Check sheet for the drawn part. Datum: minimum x, y, z corner. Units: mm. Coordinates: 2 decimals unless noted, no trailing zeros. Write each loop counter-clockwise with the first axis right and the second up, starting at its lowest first coordinate (ties: lowest second). Pieces come first, ordered by that corner, then holes. Notation, with made-up numbers: M 12.25,19.25 L 28.25,19.25 A27 cw 28.25,46.25 Z; hole C 79,42 d4. An arc over 180 degrees is marked long. Answer as CSV lines item,"result".
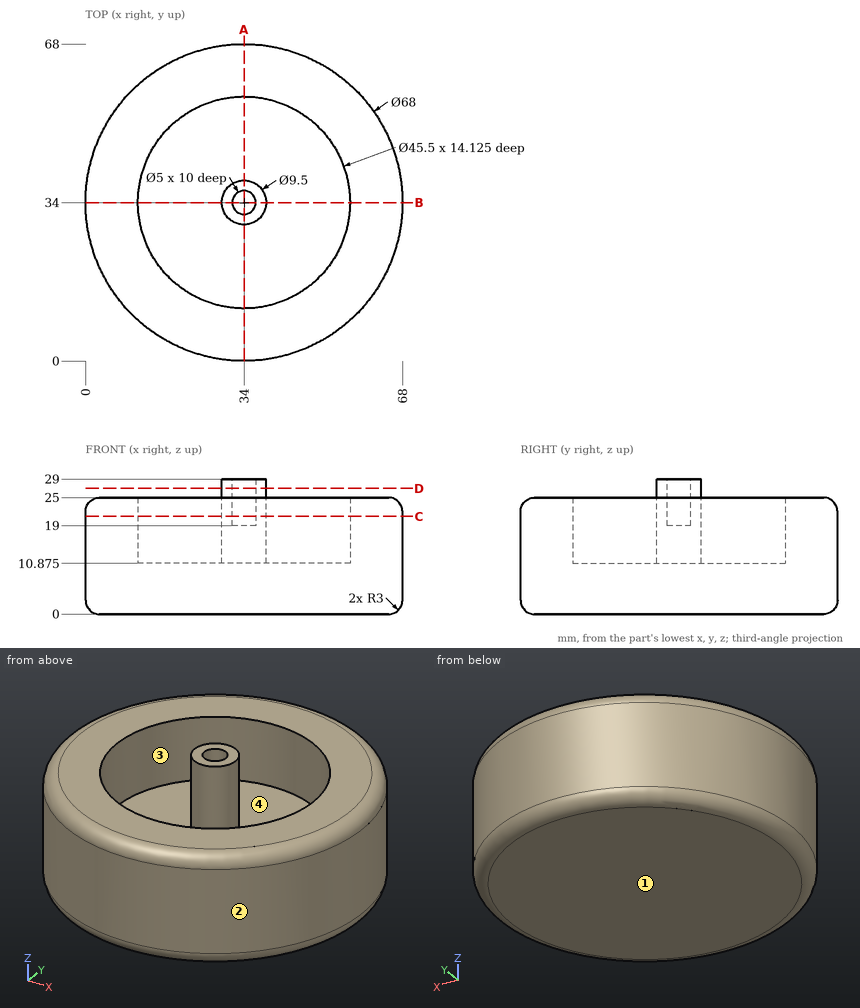
1) Depth check by flat-ended pin: P1, Ø6, axis at x = 11.5, z = 14.5, coming from the +Y side; P2, Ø8, axis at x = 49, z = 21.5, coming from the -Y side; P3, Ø12, axis at x = 49.5, z = 24.5, coming from the -Y side. Enter the tip coordinate at first touch or a pass-through.
Answer key:
P1,"stops at y = 61.85"
P2,"stops at y = 1.83"
P3,"stops at y = 1.49"
2) Section check D-D, the plane z = 27. Record the boundary of the cut face in (x, y).
Answer key:
outline,"C 34,34 d9.5; hole C 34,34 d5"
3) Mould release check, pull along Y, two halves, no side actions. Record for the marked faces 1, 2, 3 and 4: pulls with the +Y half, pulls with the -Y half, needs draft (parallel to the pull), parting line crosses it, or undercut.
Answer key:
face 1,"needs draft"
face 2,"parting line crosses it"
face 3,"undercut"
face 4,"undercut"
4) Section check C-C, the plane z = 21. Record the boundary of the cut face in (x, y), plus the area to 3 significant figures.
Answer key:
outline,"C 34,34 d68; C 34,34 d9.5; hole C 34,34 d45.5; hole C 34,34 d5"
area,"2,060 mm2"
5) Thickness scan on line 1 along Y through (x, z) = (34, 22); line 2 along X through (y, z) = (34, 15). Record the ranges inside material, lowest first.
Answer key:
line 1,"y = 0 to 11.25, 29.25 to 31.5, 36.5 to 38.75, 56.75 to 68"
line 2,"x = 0 to 11.25, 29.25 to 38.75, 56.75 to 68"
6) Section check A-A, the plane x = 34. Record the boundary of the cut face in (y, z) (3 decimals).
Answer key:
outline,"M 0,3 A3 ccw 3,0 L 65,0 A3 ccw 68,3 L 68,22 A3 ccw 65,25 L 56.75,25 L 56.75,10.875 L 38.75,10.875 L 38.75,29 L 36.5,29 L 36.5,19 L 31.5,19 L 31.5,29 L 29.25,29 L 29.25,10.875 L 11.25,10.875 L 11.25,25 L 3,25 A3 ccw 0,22 Z"
